Check sheet for the modelled part. Datum: model origin and axes. Units: mm. Coordinates: 2 decimals unless noted, no trailing zeros. Order: outer loops, then holes, each group sorted by start corner. A loop starts at its lowest first (then second) coordinate and runs counter-clockwise, first axis right, second up.
Autodesk Inventor part; units mm, degrees
ref_plane "YZ Plane" through (0, 0, 0) normal (1, 0, 0) x (0, 1, 0)
ref_plane "XZ Plane" through (0, 0, 0) normal (0, 1, 0) x (-1, 0, 0)
ref_plane "XY Plane" through (0, 0, 0) normal (0, 0, 1) x (1, 0, 0)
sketch "Sketch1" plane through (0, 0, 0) normal (0, 1, 0) x (-1, 0, 0)
  line L0 (20, 46) -> (-20, 46)
  line L1 (-20, 46) -> (-20, -46)
  line L2 (-20, -46) -> (20, -46)
  line L3 (20, -46) -> (20, 46)
  line L4 (20, 46) -> (-20, -46)
  line L5 (20, -46) -> (-20, 46)
  point P0 (0, 0)
  point P1 (0, 0)
  dimension "d9" = 92
  dimension "d10" = 40
extrude "Extrusion1" add sketch "Sketch1" along normal blind 20
fillet "Fillet5" radius 8 4 edges at (20, 20, 0) (-20, 20, 0) (20, 0, 0) (-20, 0, 0)
properties part number "battery-model-group2"
(1) Cross-section at B-B (y = 4). Enter the section's corners in (x, z), and give its area (3 significant figures).
Filled in:
outline: (-18.93, -46) - (18.93, -46) - (18.93, 46) - (-18.93, 46) - close
area: 3,480 mm2
(2) Cross-section at A-A (z = 37.5). Enter the section's corners in (x, y).
Filled in:
outline: (-20, 8) arc R8 ccw to (-12, 0) - (12, 0) arc R8 ccw to (20, 8) - (20, 12) arc R8 ccw to (12, 20) - (-12, 20) arc R8 ccw to (-20, 12) - close
(3) Go/stop test with a flat-tipped pin: P1, Ø1, axis at y = 3, z = 0.5, coming from the -X side. Record where the tip stops, or that it passes through.
Filled in:
P1: stops at x = -18.61
(4) Cross-section at C-C (x = 15). Enter the section's corners in (y, z).
Filled in:
outline: (0.58, -46) - (19.42, -46) - (19.42, 46) - (0.58, 46) - close
(5) Thickness scan on probe 1 along X at (y, z) = (7.5, 1); probe 2 along X at (y, z) = (17, 40) (3 decimals); probe 3 along Y at (x, z) = (-18, 35.5). Record the ranges inside material, lowest first.
Filled in:
probe 1: x = -19.98 to 19.98
probe 2: x = -18.245 to 18.245
probe 3: y = 2.71 to 17.29
